Autodesk Inventor part; units mm, degrees
ref_plane "YZ Plane" through (0, 0, 0) normal (1, 0, 0) x (0, 1, 0)
ref_plane "XZ Plane" through (0, 0, 0) normal (0, 1, 0) x (-1, 0, 0)
ref_plane "XY Plane" through (0, 0, 0) normal (0, 0, 1) x (1, 0, 0)
sketch "Sketch1" plane through (0, 0, 0) normal (0, 0, 1) x (1, 0, 0)
  line L0 (-12.5, 12.5) -> (12.5, 12.5)
  line L1 (12.5, 12.5) -> (12.5, -12.5)
  line L2 (12.5, -12.5) -> (-12.5, -12.5)
  line L3 (-12.5, -12.5) -> (-12.5, 12.5)
  circle A0 centre (0, 0) radius 8
  point P0 (0, 12.5)
  point P1 (-12.5, 0)
  dimension "d0" = 25
  dimension "d2" = 16
extrude "Extrusion1" add sketch "Sketch1" along normal blind 3
sketch "Sketch2" plane through (0, 0, 3) normal (0, 0, 1) x (1, 0, 0)
  circle A0 centre (0, 0) radius 8
  line L0 (12.5, 12.5) -> (-12.5, 12.5)
  line L1 (-12.5, 12.5) -> (-12.5, -12.5)
  line L2 (-12.5, -12.5) -> (12.5, -12.5)
  line L3 (12.5, -12.5) -> (12.5, 12.5)
  circle A1 centre (0, 0) radius 6
  dimension "d5" = 12
extrude "Extrusion2" add sketch "Sketch2" along normal blind 6 contours A0 | L3 L2 L1 L0
sketch "Sketch3" plane through (0, 0, 9) normal (0, 0, 1) x (1, 0, 0)
  line L0 (12.5, 12.5) -> (-12.5, 12.5)
  line L1 (-12.5, 12.5) -> (-12.5, -12.5)
  line L2 (-12.5, -12.5) -> (12.5, -12.5)
  line L3 (12.5, -12.5) -> (12.5, 12.5)
  circle A0 centre (0, 0) radius 8
extrude "Extrusion3" add sketch "Sketch3" along normal blind 3
sketch "Sketch4" plane through (0, 0, 12) normal (0, 0, 1) x (1, 0, 0)
  circle A0 centre (0, 0) radius 8
  line L0 (-12.5, 12.5) -> (-12.5, -12.5)
  line L1 (-12.5, 0.75) -> (12.5, 0.75)
  line L2 (12.5, 0.75) -> (12.5, -12.5)
  line L3 (12.5, -12.5) -> (-12.5, -12.5)
  line L4 (-12.5, -12.5) -> (-12.5, 0.75)
  dimension "d11" = 0.75
extrude "Extrusion4" cut sketch "Sketch4" against normal through all contours A0 L1 | A0 L1 L2 L3 L0 picked at (-1.088, -1.9346)
sketch "Sketch5" plane through (-12.5, 12.5, 0) normal (0, 1, 0) x (1, 0, 0)
  line L0 (0, 0) -> (0, -12)
  line L1 (25, 0) -> (25, -12)
  circle A0 centre (3.5, -6) radius 1.75
  circle A1 centre (21.5, -6) radius 1.75
  point P0 (12.5, 0)
  point P1 (25, -6)
  point P2 (0, -6)
  dimension "d14" = 3.5
  dimension "d16" = 3.5
  dimension "d17" = 3.5
extrude "Extrusion5" cut sketch "Sketch5" against normal through all
sketch "Sketch6" plane through (-12.5, 12.5, 0) normal (0, 1, 0) x (1, 0, 0)
  circle A0 centre (3.5, -6) radius 1.75
  circle A1 centre (21.5, -6) radius 1.75
  circle A2 centre (3.5, -6) radius 3
  circle A3 centre (21.5, -6) radius 3
  point P0 (12.5, 0)
  dimension "d20" = 6
  dimension "d22" = 6
extrude "Extrusion6" cut sketch "Sketch6" against normal blind 3
fillet "Fillet1" radius 2.5 2 edges at (-12.5, 12.5, 6) (12.5, 12.5, 6)
properties part number "e3d mount"
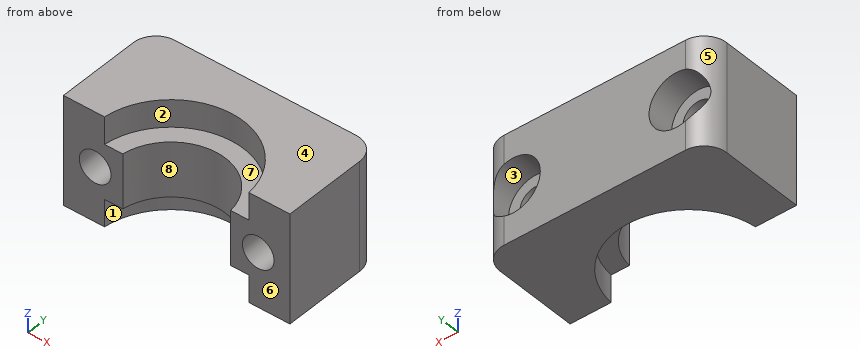
Verification items for the finished model (mm, model axes). Face numbers are marked on the shaded views. A direction names the side the tool comes from. Give positions to 0.01 mm unless a question says otherwise; leave off trailing zeros. Loops run counter-clockwise (first coordinate to the right, second up) from the corner with the lowest first, then second, coordinate; pieces in that order, holes last. Notation, with made-up numbers: (52, -24.75) - (74, -24.75) arc R14 ccw to (74, 1.25) - close; hole circle Ø9 at (-7, 70.25). An arc over 180 degrees is marked (long way). Write item = value, one per line. Start each with the question number.
Q1. Tool access check on the marked faces 1, 2, 3 and 4. Record the directions out of +Z, -Z, +X, -X, +Y, -Y that give a thin tool (end or side, any length) a straight path to the whole face; none if there is none.
Q2. Cross-section at A-A, the plane x = -9. Enter the section's corners in (y, z).
Q3. Cross-section at C-C, the plane z = 6. Enter the section's corners in (x, y).
Q4. Thickness scan on line 1 (X direction, y = 6.5, z = 6); line 2 (Z direction, x = 9, y = 10.85); line 3 (X direction, y = 10.9, z = 6). Record the ranges inside material, lowest first.
Q5. Mould release check, pull along X, two halves, no side actions. Record for the marked faces 5, 6, 7 and 8: released by +X, released by -X, zero draft, split by the parting line, or undercut.
Q6. Cross-section at D-D, the plane z = 2.5. Enter the section's corners in (x, y), and give its area (3 significant figures).
Q7. Depth check by flat-ended pin: P1, Ø2, axis at x = 9, z = 6, coming from the +Y side; P2, Ø5, axis at x = 9, z = 6, coming from the +Y side; P3, Ø5, axis at x = -9, z = 7.5, coming from the +Y side; P4, Ø3.5, axis at x = 3.5, y = 3.5, coming from the -Z side. Enter the tip coordinate at first touch or a pass-through.
Q8. Cross-section at B-B, the plane y = 3.25. Enter the section's corners in (x, z), and give its area (3 significant figures).
Answer key:
q1.face_1 = -Z, -Y
q1.face_2 = +Z, -Y
q1.face_3 = +Y
q1.face_4 = +Z, +X, -X, +Y, -Y
q2.outline = (0.75, 0) - (12.5, 0) - (12.5, 3) - (9.5, 3) - (9.5, 4.25) - (0.75, 4.25) - close; (0.75, 7.75) - (9.5, 7.75) - (9.5, 9) - (12.5, 9) - (12.5, 12) - (0.75, 12) - close
q3.outline = (-12.5, 0.75) - (-10.75, 0.75) - (-10.75, 9.5) - (-12, 9.5) - (-12, 11.5) arc R2.5 ccw to (-12.5, 10) - close; (-7.25, 0.75) - (-5.95, 0.75) arc R6 cw to (5.95, 0.75) - (7.25, 0.75) - (7.25, 9.5) - (6, 9.5) - (6, 12.5) - (-6, 12.5) - (-6, 9.5) - (-7.25, 9.5) - close; (10.75, 0.75) - (12.5, 0.75) - (12.5, 10) arc R2.5 ccw to (12, 11.5) - (12, 9.5) - (10.75, 9.5) - close
q4.line_1 = -12.5 to -10.75, -7.25 to 7.25, 10.75 to 12.5
q4.line_2 = 0 to 3, 9 to 12
q4.line_3 = -12.33 to -12, -6 to 6, 12 to 12.33
q5.face_5 = released by -X
q5.face_6 = zero draft
q5.face_7 = undercut
q5.face_8 = undercut
q6.outline = (-12.5, 0.75) - (-7.96, 0.75) arc R8 cw to (7.96, 0.75) - (12.5, 0.75) - (12.5, 10) arc R2.5 ccw to (10, 12.5) - (-10, 12.5) arc R2.5 ccw to (-12.5, 10) - close
q6.area = 203 mm^2
q7.P1 = through
q7.P2 = 9.5
q7.P3 = 12.5
q7.P4 = 3
q8.outline = (-12.5, 0) - (-7.31, 0) - (-7.31, 3) - (-5.04, 3) - (-5.04, 9) - (-7.31, 9) - (-7.31, 12) - (-12.5, 12) - close; (5.04, 3) - (7.31, 3) - (7.31, 0) - (12.5, 0) - (12.5, 12) - (7.31, 12) - (7.31, 9) - (5.04, 9) - close; hole circle Ø3.5 at (-9, 6); hole circle Ø3.5 at (9, 6)
q8.area = 133 mm^2
